from build123d import *

# Parameters (mm, degrees)
BOSS_EXTRUDE1_DEPTH      = 10
BOSS_EXTRUDE1_DEPTH_BACK = 10
CUT_EXTRUDE1_DEPTH       = 10
CUT_EXTRUDE1_DEPTH_BACK  = 10


with BuildPart() as part:
    # Sketch13 → Boss-Extrude1 (new body, two sides)
    with BuildSketch(Plane(origin=(-31.8, 0, 0), x_dir=(0, 0, -1), z_dir=(1, 0, 0))) as boss_extrude1_sk:
        with BuildLine():
            Line((6.746523488, 9.38), (3.731523488, 14.602133185))
            Line((3.731523488, 14.602133185), (8.392906101, 23.38137644))
            Line((8.392906101, 23.38137644), (13.476604558, 23.38137644))
            ThreePointArc((13.476604558, 23.38137644), (15.597924901, 22.502696784), (16.476604558, 20.38137644))
            Line((16.476604558, 20.38137644), (16.476604558, 9.38))
            Line((16.476604558, 9.38), (6.746523488, 9.38))
        make_face()
    extrude(amount=BOSS_EXTRUDE1_DEPTH)
    extrude(boss_extrude1_sk.sketch, amount=-BOSS_EXTRUDE1_DEPTH_BACK)

    # Sketch15 → Cut-Extrude1 (cut, two sides)
    with BuildSketch(Plane(origin=(-31.8, 0, 0), x_dir=(0, 0, -1), z_dir=(1, 0, 0))) as cut_extrude1_sk:
        Polygon((10.184407321, 19.178855838), (9.360685737, 17.752128204), (11.525749246, 16.502128204), (8.497418172, 11.256904921), (6.332354663, 12.506904921), (5.636779377, 11.302133185), (3.617891994, 14.798948707), (6.332354663, 19.500535964), (7.368827308, 18.902128204), (8.192548892, 20.328855838), align=None)
    extrude(amount=CUT_EXTRUDE1_DEPTH, mode=Mode.SUBTRACT)
    extrude(cut_extrude1_sk.sketch, amount=-CUT_EXTRUDE1_DEPTH_BACK, mode=Mode.SUBTRACT)


solid = part.part
Geometry: final body of the model. Coordinates: model frame, mm. A direction names the side the tool comes from. Give positions to 0.01 mm unless a question says otherwise; leave off trailing zeros. Order: outer loops, then holes, each group sorted by start corner. A loop starts at its lowest first (then second) coordinate and runs counter-clockwise, first axis right, second up. Notation, with made-up numbers: (-9, 21.25) -> (29, 21.25) arc R25 ccw to (29, 55.25) -> close; hole circle Ø1 at (40.25, 37.5). An arc over 180 degrees is marked (long way). Put each result on its own line as item: value.
Q1. Material intervals for L1, parallel to Y at x = -27.25, z = -10; L2, parallel to Z at x = -26.75, y = 12.75; L3, parallel to Y at x = -40.25, z = -9.5, sorted ascending.
Here are the results:
L1: y = 9.38 to 13.86, 17.38 to 18.86, 19.29 to 23.38
L2: z = -16.48 to -9.36
L3: y = 9.38 to 12.99, 17.67 to 17.99, 19.57 to 23.38
Q2. Pin query (flat end, axial travel): pin 1 (4 mm diameter, centred on x = -28.5, y = 15, fed in from +Z); pin 2 (6 mm diameter, centred on y = 19.5, z = -8.5, fed in from +X); pin 3 (2 mm diameter, centred on x = -26.5, z = -15, fed in from +Y). Return the tip coordinate at first contact, or that it passes through.
Here are the results:
pin 1: stops at z = -9.5
pin 2: stops at x = -21.8
pin 3: stops at y = 23.34
Q3. Section D-D, the plane y = 22. Return loops of the section in (x, z).
Here are the results:
outline: (-41.8, -16) -> (-21.8, -16) -> (-21.8, -7.66) -> (-41.8, -7.66) -> close
Q4. Reachability of faces 1 (the face through (-31.94, 19.206, -6.843)), 2 (the face through (-31.7, 22.5, -15.6)), 3 (the face through (-31.94, 19.606, -7.775)) from +Z, -Z, +X, -X, +Y, -Y: full face, straight path, thin tool, end or side. Return the list, or none.
Here are the results:
face 1: +Z, +X, -X
face 2: -Z, +X, -X, +Y
face 3: +X, -X
Q5. Section B-B, the plane x = -33.5. Return loops of the section in (y, z), then the cut area to 3 significant figures.
Here are the results:
outline: (9.38, -16.48) -> (20.38, -16.48) arc R3 ccw to (23.38, -13.48) -> (23.38, -8.39) -> (19.5, -6.33) -> (18.9, -7.37) -> (20.33, -8.19) -> (19.18, -10.18) -> (17.75, -9.36) -> (16.5, -11.53) -> (11.26, -8.5) -> (12.51, -6.33) -> (11.3, -5.64) -> (9.38, -6.75) -> close
area: 107 mm^2
Q6. Section A-A, the plane z = -9.75. Return loops of the section in (x, y).
Here are the results:
outline: (-41.8, 9.38) -> (-21.8, 9.38) -> (-21.8, 13.43) -> (-41.8, 13.43) -> close; (-41.8, 17.53) -> (-21.8, 17.53) -> (-21.8, 18.43) -> (-41.8, 18.43) -> close; (-41.8, 19.43) -> (-21.8, 19.43) -> (-21.8, 23.38) -> (-41.8, 23.38) -> close
Q7. Section C-C, the plane y = 15.5. Return loops of the section in (x, z), then the cut area to 3 significant figures.
Here are the results:
outline: (-41.8, -16.48) -> (-21.8, -16.48) -> (-21.8, -10.95) -> (-41.8, -10.95) -> close
area: 111 mm^2
Q8. Draft query along Y for faces 4 (the face through (-31.94, 17.136, -10.428)), 5 (the face through (-32, 23.381, -11)), 6 (the face through (-21.8, 16, -12)). Return one class per face: released by +Y, released by -Y, zero draft, split by the parting line, or undercut.
Here are the results:
face 4: undercut
face 5: released by +Y
face 6: zero draft
